The listing builds one solid part. Answer for the finished solid, in the listing's coordinates (mm). Round coordinates to 2 decimals unless told otherwise and drop trailing zeros. Order: outer loops, then holes, each group sorted by start corner. A loop starts at its lowest first (then second) coordinate and runs counter-clockwise, first axis right, second up. Notation, with made-up numbers: (30, 88.5) -> (48, 88.5) arc R30 cw to (48, 120.5) -> close; hole circle Ø10 at (10, 64.25). An arc over 180 degrees is marked (long way). Answer in a Markdown table with one row per item. Add a question column.
```python
from build123d import *

# Parameters (mm, degrees)
SKETCH1_R           = 1.5
SKETCH1_R_2         = 2
SKETCH1_W           = 9
SKETCH1_H           = 13.2
BOSS_EXTRUDE1_DEPTH = 4
SKETCH2_R           = 1.5
CUT_EXTRUDE1_DEPTH  = 4


with BuildPart() as part:
    # Sketch1 → Boss-Extrude1 (new body)
    with BuildSketch(Plane(origin=(0, 0, 0), x_dir=(1, 0, 0), z_dir=(0, 1, 0))):
        with BuildLine():
            Line((-72, 110), (-48, 110))
            ThreePointArc((-48, 110), (-45.878679656, 109.121320344), (-45, 107))
            Line((-45, 107), (-45, 100))
            Line((-45, 100), (-74.819077862, 18.072756904))
            ThreePointArc((-74.819077862, 18.072756904), (-74.954423259, 17.567641007), (-75, 17.046696474))
            Line((-75, 17.046696474), (-75, -127))
            ThreePointArc((-75, -127), (-74.121320344, -129.121320344), (-72, -130))
            Line((-72, -130), (72, -130))
            ThreePointArc((72, -130), (74.121320344, -129.121320344), (75, -127))
            Line((75, -127), (75, 17.046696474))
            ThreePointArc((75, 17.046696474), (74.954423259, 17.567641007), (74.819077862, 18.072756904))
            Line((74.819077862, 18.072756904), (45, 100))
            Line((45, 100), (45, 107))
            ThreePointArc((45, 107), (45.878679656, 109.121320344), (48, 110))
            Line((48, 110), (72, 110))
            ThreePointArc((72, 110), (74.121320344, 110.878679656), (75, 113))
            Line((75, 113), (75, 127))
            ThreePointArc((75, 127), (74.121320344, 129.121320344), (72, 130))
            Line((72, 130), (-72, 130))
            ThreePointArc((-72, 130), (-74.121320344, 129.121320344), (-75, 127))
            Line((-75, 127), (-75, 113))
            ThreePointArc((-75, 113), (-74.121320344, 110.878679656), (-72, 110))
        make_face()
        with Locations((20, 90)):
            Circle(SKETCH1_R, mode=Mode.SUBTRACT)
        with Locations((-20, 90)):
            Circle(SKETCH1_R, mode=Mode.SUBTRACT)
        with Locations((-66.538461538, -72)):
            Circle(SKETCH1_R_2, mode=Mode.SUBTRACT)
        with Locations((-66.538461538, -88)):
            Circle(SKETCH1_R_2, mode=Mode.SUBTRACT)
        with Locations((-52.538461538, -72)):
            Circle(SKETCH1_R_2, mode=Mode.SUBTRACT)
        with Locations((-52.538461538, -88)):
            Circle(SKETCH1_R_2, mode=Mode.SUBTRACT)
        with Locations((52.538461538, -88)):
            Circle(SKETCH1_R_2, mode=Mode.SUBTRACT)
        with Locations((66.538461538, -88)):
            Circle(SKETCH1_R_2, mode=Mode.SUBTRACT)
        with Locations((66.538461538, -72)):
            Circle(SKETCH1_R_2, mode=Mode.SUBTRACT)
        with Locations((52.538461538, -72)):
            Circle(SKETCH1_R_2, mode=Mode.SUBTRACT)
        with Locations((-18.75, -58.75)):
            Circle(SKETCH1_R, mode=Mode.SUBTRACT)
        with BuildLine():
            Line((-70.5, 121.5), (-60.5, 121.5))
            ThreePointArc((-60.5, 121.5), (-59, 120), (-60.5, 118.5))
            Line((-60.5, 118.5), (-70.5, 118.5))
            ThreePointArc((-70.5, 118.5), (-72, 120), (-70.5, 121.5))
        make_face(mode=Mode.SUBTRACT)
        with BuildLine():
            Line((-19, -12.5), (19, -12.5))
            ThreePointArc((19, -12.5), (19.707106781, -12.792893219), (20, -13.5))
            Line((20, -13.5), (20, -16.5))
            ThreePointArc((20, -16.5), (19.707106781, -17.207106781), (19, -17.5))
            Line((19, -17.5), (-19, -17.5))
            ThreePointArc((-19, -17.5), (-19.707106781, -17.207106781), (-20, -16.5))
            Line((-20, -16.5), (-20, -13.5))
            ThreePointArc((-20, -13.5), (-19.707106781, -12.792893219), (-19, -12.5))
        make_face(mode=Mode.SUBTRACT)
        with BuildLine():
            Line((-15, 121.5), (-5, 121.5))
            ThreePointArc((-5, 121.5), (-3.5, 120), (-5, 118.5))
            Line((-5, 118.5), (-15, 118.5))
            ThreePointArc((-15, 118.5), (-16.5, 120), (-15, 121.5))
        make_face(mode=Mode.SUBTRACT)
        with Locations((55, 5)):
            Rectangle(SKETCH1_W, SKETCH1_H, mode=Mode.SUBTRACT)
        with BuildLine():
            Line((-50.5, 121.5), (-40.5, 121.5))
            ThreePointArc((-40.5, 121.5), (-39, 120), (-40.5, 118.5))
            Line((-40.5, 118.5), (-50.5, 118.5))
            ThreePointArc((-50.5, 118.5), (-52, 120), (-50.5, 121.5))
        make_face(mode=Mode.SUBTRACT)
        with BuildLine():
            Line((5, 118.5), (15, 118.5))
            ThreePointArc((15, 118.5), (16.5, 120), (15, 121.5))
            Line((15, 121.5), (5, 121.5))
            ThreePointArc((5, 121.5), (3.5, 120), (5, 118.5))
        make_face(mode=Mode.SUBTRACT)
        with BuildLine():
            Line((19, 102.5), (-19, 102.5))
            ThreePointArc((-19, 102.5), (-19.707106781, 102.792893219), (-20, 103.5))
            Line((-20, 103.5), (-20, 106.5))
            ThreePointArc((-20, 106.5), (-19.707106781, 107.207106781), (-19, 107.5))
            Line((-19, 107.5), (19, 107.5))
            ThreePointArc((19, 107.5), (19.707106781, 107.207106781), (20, 106.5))
            Line((20, 106.5), (20, 103.5))
            ThreePointArc((20, 103.5), (19.707106781, 102.792893219), (19, 102.5))
        make_face(mode=Mode.SUBTRACT)
        with BuildLine():
            Line((-17.25, -21.25), (-17.25, -23.25))
            ThreePointArc((-17.25, -23.25), (-18.75, -24.75), (-20.25, -23.25))
            Line((-20.25, -23.25), (-20.25, -21.25))
            ThreePointArc((-20.25, -21.25), (-18.75, -19.75), (-17.25, -21.25))
        make_face(mode=Mode.SUBTRACT)
        with BuildLine():
            Line((18.75, -60.25), (17.75, -60.25))
            ThreePointArc((17.75, -60.25), (16.25, -58.75), (17.75, -57.25))
            Line((17.75, -57.25), (18.75, -57.25))
            ThreePointArc((18.75, -57.25), (20.25, -58.75), (18.75, -60.25))
        make_face(mode=Mode.SUBTRACT)
        with BuildLine():
            Line((19.810660172, -22.310660172), (16.275126266, -25.846194078))
            ThreePointArc((16.275126266, -25.846194078), (14.153805922, -25.846194078), (14.153805922, -23.724873734))
            Line((14.153805922, -23.724873734), (17.689339828, -20.189339828))
            ThreePointArc((17.689339828, -20.189339828), (19.810660172, -20.189339828), (19.810660172, -22.310660172))
        make_face(mode=Mode.SUBTRACT)
        with BuildLine():
            Line((50.5, 121.5), (40.5, 121.5))
            ThreePointArc((40.5, 121.5), (39, 120), (40.5, 118.5))
            Line((40.5, 118.5), (50.5, 118.5))
            ThreePointArc((50.5, 118.5), (52, 120), (50.5, 121.5))
        make_face(mode=Mode.SUBTRACT)
        with BuildLine():
            Line((60.5, 118.5), (70.5, 118.5))
            ThreePointArc((70.5, 118.5), (72, 120), (70.5, 121.5))
            Line((70.5, 121.5), (60.5, 121.5))
            ThreePointArc((60.5, 121.5), (59, 120), (60.5, 118.5))
        make_face(mode=Mode.SUBTRACT)
    extrude(amount=BOSS_EXTRUDE1_DEPTH)

    # Sketch2 → Cut-Extrude1 (cut)
    with BuildSketch(Plane(origin=(0, 4, 0), x_dir=(1, 0, 0), z_dir=(0, 1, 0))):
        with Locations((-71, -126)):
            Circle(SKETCH2_R)
        with Locations((-71, 16.870369494)):
            Circle(SKETCH2_R)
        with Locations((-71, 114)):
            Circle(SKETCH2_R)
        with Locations((-71, 126)):
            Circle(SKETCH2_R)
        with Locations((71, 16.870369494)):
            Circle(SKETCH2_R)
        with Locations((71, -126)):
            Circle(SKETCH2_R)
        with Locations((71, 114)):
            Circle(SKETCH2_R)
        with Locations((71, 126)):
            Circle(SKETCH2_R)
        with Locations((-40, 70)):
            Circle(SKETCH2_R)
        with Locations((40, 70)):
            Circle(SKETCH2_R)
        with BuildLine():
            Line((-20, -71), (-17, -71))
            ThreePointArc((-17, -71), (-16.292893219, -71.292893219), (-16, -72))
            Line((-16, -72), (-16, -88))
            ThreePointArc((-16, -88), (-16.292893219, -88.707106781), (-17, -89))
            Line((-17, -89), (-20, -89))
            ThreePointArc((-20, -89), (-20.707106781, -88.707106781), (-21, -88))
            Line((-21, -88), (-21, -72))
            ThreePointArc((-21, -72), (-20.707106781, -71.292893219), (-20, -71))
        make_face()
        with BuildLine():
            Line((-26.5, -28.5), (-23.5, -28.5))
            ThreePointArc((-23.5, -28.5), (-22.792893219, -28.792893219), (-22.5, -29.5))
            Line((-22.5, -29.5), (-22.5, -37.5))
            ThreePointArc((-22.5, -37.5), (-22.792893219, -38.207106781), (-23.5, -38.5))
            Line((-23.5, -38.5), (-26.5, -38.5))
            ThreePointArc((-26.5, -38.5), (-27.207106781, -38.207106781), (-27.5, -37.5))
            Line((-27.5, -37.5), (-27.5, -29.5))
            ThreePointArc((-27.5, -29.5), (-27.207106781, -28.792893219), (-26.5, -28.5))
        make_face()
        with BuildLine():
            Line((26.5, -38.5), (23.5, -38.5))
            ThreePointArc((23.5, -38.5), (22.792893219, -38.207106781), (22.5, -37.5))
            Line((22.5, -37.5), (22.5, -29.5))
            ThreePointArc((22.5, -29.5), (22.792893219, -28.792893219), (23.5, -28.5))
            Line((23.5, -28.5), (26.5, -28.5))
            ThreePointArc((26.5, -28.5), (27.207106781, -28.792893219), (27.5, -29.5))
            Line((27.5, -29.5), (27.5, -37.5))
            ThreePointArc((27.5, -37.5), (27.207106781, -38.207106781), (26.5, -38.5))
        make_face()
        with BuildLine():
            Line((16, -72), (16, -88))
            ThreePointArc((16, -88), (16.292893219, -88.707106781), (17, -89))
            Line((17, -89), (20, -89))
            ThreePointArc((20, -89), (20.707106781, -88.707106781), (21, -88))
            Line((21, -88), (21, -72))
            ThreePointArc((21, -72), (20.707106781, -71.292893219), (20, -71))
            Line((20, -71), (17, -71))
            ThreePointArc((17, -71), (16.292893219, -71.292893219), (16, -72))
        make_face()
    extrude(amount=-CUT_EXTRUDE1_DEPTH, mode=Mode.SUBTRACT)


solid = part.part
```
Item 1: For a pull along Z with two mould halves and no side action, classify faces 1 (the face through (60.12, 1.97, -58.46)), 2 (the face through (-59.7, 1.97, -59.61)), 3 (the face through (-1, 0, -2)) as released by +Z, released by -Z, zero draft, split by the parting line, or undercut.
Item 2: A flat-ended cylindrical pin translates along its axis: P1, Ø1.8, axis at x = -20, z = -90, coming from the +Y side. Find the tip coordinate at first contact, or state that the pin passes through.
Item 3: The part is cut by section A-A, the plane z = -1.5. Give the vertices of the cut face in (x, y), and give its area (3 significant figures).
Item 4: The part is cut by section C-C, the plane y = 2.1. State how many separate pieces and enclosed holes the cut face has, and give its area (3 significant figures).
Item 5: The part is cut by section B-B, the plane x = -11.5. Give the vertices of the cut face in (y, z), and give its area (3 significant figures).
Item 6: Find the intervals of material crossed by probe 1 along Z at (x, y) = (5, 2.5); probe 2 along X at (y, z) = (2.5, 84); probe 3 along X at (y, z) = (0.35, 30.5), in increasing order. Write a range as [from, to].
Item 7: The part is cut by section D-D, the plane z = -44.5. Give the vertices of the cut face in (x, y).
Resolved:
| question | item | result |
|---|---|---|
| 1 | face 1 | undercut |
| 1 | face 2 | undercut |
| 1 | face 3 | zero draft |
| 2 | P1 | through |
| 3 | outline | (-75, 0) -> (50.5, 0) -> (50.5, 4) -> (-75, 4) -> close; (59.5, 0) -> (75, 0) -> (75, 4) -> (59.5, 4) -> close |
| 3 | area | 564 mm2 |
| 4 | separate pieces | 1 |
| 4 | enclosed holes | 37 |
| 4 | area | 34,700 mm2 |
| 5 | outline | (0, -130) -> (4, -130) -> (4, -121.5) -> (0, -121.5) -> close; (0, -118.5) -> (4, -118.5) -> (4, -107.5) -> (0, -107.5) -> close; (0, -102.5) -> (4, -102.5) -> (4, 12.5) -> (0, 12.5) -> close; (0, 17.5) -> (4, 17.5) -> (4, 130) -> (0, 130) -> close |
| 5 | area | 988 mm2 |
| 6 | probe 1 | [-130, -121.5], [-118.5, -107.5], [-102.5, 12.5], [17.5, 130] |
| 6 | probe 2 | [-75, -21], [-16, 16], [21, 75] |
| 6 | probe 3 | [-75, -27.5], [-22.5, 22.5], [27.5, 75] |
| 7 | outline | (-65.2, 0) -> (65.2, 0) -> (65.2, 4) -> (-65.2, 4) -> close |
